Solid Edge part; units mm, degrees
sketch "Sketch1" plane through (0, 0, 0) normal (0, -1, 0) x (1, 0, 0)
  line L0 (90, 20) -> (90, 45)
  line L1 (90, 45) -> (85, 45)
  line L2 (85, 45) -> (60, 20)
  line L3 (35, 45) -> (60, 20)
  line L4 (30, 45) -> (35, 45)
  line L5 (30, 20) -> (30, 45)
  line L6 (0, 20) -> (30, 20)
  line L7 (0, 0) -> (0, 20)
  line L8 (0, 0) -> (120, 0)
  line L9 (120, 0) -> (120, 20)
  line L10 (120, 20) -> (90, 20)
extrude "Protrusion1" add sketch "Sketch1" against normal blind 45
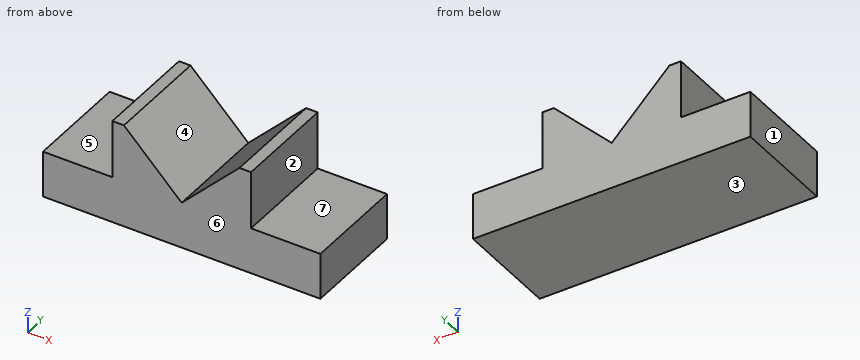
Work out the finished part from the listing and answer in its coordinate system (mm). Face numbers are marked on the shaded views. A direction names the side the tool comes from. Give positions to 0.01 mm unless a question says otherwise; leave off trailing zeros. Loops run counter-clockwise (first coordinate to the right, second up) from the corner with the lowest first, then second, coordinate; pieces in that order, holes last. Notation, with made-up numbers: (29.25, 20.5) -> (78.25, 20.5) arc R17 cw to (78.25, 31.5) -> close; hole circle Ø1 at (-5, -32). An arc over 180 degrees is marked (long way). Put each result on its own line as item: value. Start each with the question number.
Item 1: The part is cut by section C-C (x = 25). Give the vertices of the cut face in (y, z).
Item 2: The part is cut by section B-B (y = 33). Give the vertices of the cut face in (x, z), then the cut area to 4 significant figures.
Item 3: The part is cut by section A-A (z = 35). Give the vertices of the cut face in (x, y).
Item 4: The mould has two halves that part along X. Classify the marked faces 1, 2, 3 and 4: released by +X, released by -X, zero draft, split by the parting line, or undercut.
Item 5: The part is cut by section D-D (z = 28). Give the vertices of the cut face in (x, y).
Item 6: Find the intervals of material crossed by L1, parallel to Z at x = 5.5, y = 8; L2, parallel to X at y = 35, z = 23; L3, parallel to X at y = 27, z = 23.5, in increasing order. Write a range as [from, to].
Item 7: Each of these flat-tipped pins is pushed along its axis until it touches: P1, Ø2, axis at y = 15.5, z = 17.5, coming from the -X side; P2, Ø7.5, axis at y = 28.5, z = 36.5, coming from the -X side; P3, Ø12, axis at y = 20, z = 36, coming from the +X side; P4, Ø10, axis at x = 19, y = 33.5, coming from the +Z side. Where does it stop, or does it pass through?
Item 8: Which of the six approach directions +Z, -Z, +X, -X, +Y, -Y give full straight-line access (tool end or side, diameter ignored) to the marked faces 5, 6 and 7?
Answers below:
1. outline: (0, 0) -> (45, 0) -> (45, 20) -> (0, 20) -> close
2. outline: (0, 0) -> (120, 0) -> (120, 20) -> (90, 20) -> (90, 45) -> (85, 45) -> (60, 20) -> (35, 45) -> (30, 45) -> (30, 20) -> (0, 20) -> close
2. area: 3,275 mm2
3. outline: (30, 0) -> (45, 0) -> (45, 45) -> (30, 45) -> close; (75, 0) -> (90, 0) -> (90, 45) -> (75, 45) -> close
4. face 1: released by -X
4. face 2: released by +X
4. face 3: zero draft
4. face 4: undercut
5. outline: (30, 0) -> (52, 0) -> (52, 45) -> (30, 45) -> close; (68, 0) -> (90, 0) -> (90, 45) -> (68, 45) -> close
6. L1: [0, 20]
6. L2: [30, 57], [63, 90]
6. L3: [30, 56.5], [63.5, 90]
7. P1: x = 0
7. P2: x = 30
7. P3: x = 90
7. P4: z = 20
8. face 5: +Z, -X, +Y, -Y
8. face 6: +Z, -Z, +X, -X, -Y
8. face 7: +Z, +X, +Y, -Y
